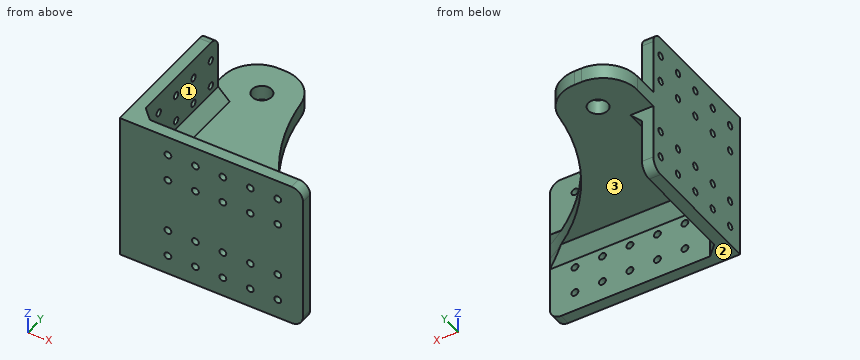
```python
from build123d import *

# Parameters (mm, degrees)
BOSS_EXTRU_1_DEPTH           = 65
ESQUISSE2_W                  = 80
ESQUISSE2_H                  = 6.5
BOSS_EXTRU_2_DEPTH           = 81
ENL_V_MAT_EXTRU_1_DEPTH      = 123.776473724
ENL_V_MAT_EXTRU_1_DEPTH_BACK = 123.776473724
CONG_1_R                     = 15
ENL_V_MAT_EXTRU_2_DEPTH      = 123.776473724
ENL_V_MAT_EXTRU_2_DEPTH_BACK = 123.776473724
ESQUISSE4_R                  = 4.25
CHANFREIN1_SIZE              = 5
ENL_V_MAT_EXTRU_3_DEPTH      = 135.242318216
ENL_V_MAT_EXTRU_3_DEPTH_BACK = 135.242318216
ESQUISSE5_R                  = 1.5
CONG_2_R                     = 5
ENL_V_MAT_EXTRU_4_DEPTH      = 135.242318216
ENL_V_MAT_EXTRU_4_DEPTH_BACK = 135.242318216
ESQUISSE6_R                  = 1.5


with BuildPart() as part:
    # Esquisse1 → Boss.-Extru.1 (new body)
    with BuildSketch(Plane.XY):
        Polygon((0, 0), (80, 0), (80, 5), (5, 5), (5, 60), (0, 60), align=None)
    extrude(amount=BOSS_EXTRU_1_DEPTH)

    # Esquisse2 → Boss.-Extru.2 (add)
    with BuildSketch(Plane(origin=(0, 5, 0), x_dir=(1, 0, 0), z_dir=(0, 1, 0))):
        with Locations((40, -32.5)):
            Rectangle(ESQUISSE2_W, ESQUISSE2_H)
    extrude(amount=BOSS_EXTRU_2_DEPTH)

    # Esquisse3 → Enlèv. mat.-Extru.1 (cut, two sides: drawn at the far end of the back side and taken through both)
    with BuildSketch(Plane.XY.offset(35.75).offset(-ENL_V_MAT_EXTRU_1_DEPTH_BACK)):
        with BuildLine():
            Line((32, 86), (80, 86))
            Line((80, 86), (80, 5))
            ThreePointArc((80, 5), (44.901203691, 38.922935521), (32, 86))
        make_face()
    extrude(amount=ENL_V_MAT_EXTRU_1_DEPTH + ENL_V_MAT_EXTRU_1_DEPTH_BACK, mode=Mode.SUBTRACT)

    # Congé1
    cong_1_edges = [part.edges().sort_by_distance(p)[0] for p in [
        (0, 86, 32.5),
        (32, 86, 32.5),
    ]]
    fillet(cong_1_edges, radius=CONG_1_R)

    # Esquisse4 → Enlèv. mat.-Extru.2 (cut, two sides: drawn at the far end of the back side and taken through both)
    with BuildSketch(Plane.XY.offset(35.75).offset(-ENL_V_MAT_EXTRU_2_DEPTH_BACK)):
        with Locations((17.5, 70.5)):
            Circle(ESQUISSE4_R)
    extrude(amount=ENL_V_MAT_EXTRU_2_DEPTH + ENL_V_MAT_EXTRU_2_DEPTH_BACK, mode=Mode.SUBTRACT)

    # Chanfrein1
    # the kernel refuses this chamfer: 5 mm, written as the material it adds along each edge
    with BuildSketch(Plane(origin=(8.333333333, 8.333333333, 39.083333333), x_dir=(0, 0.7071067811865474, -0.7071067811865476), z_dir=(-0.5773502691896261, -0.5773502691896257, -0.5773502691896255))) as chanfrein1_piece_1_section:
        Polygon((-3.535533906, 2.041241452), (3.535533906, 2.041241452), (0, -4.082482905), align=None)
    chanfrein1_piece_1 = extrude(amount=6.350852961, mode=Mode.PRIVATE)
    chanfrein1_piece_1 = split(chanfrein1_piece_1, bisect_by=Plane(origin=(5, 5, 35.75), z_dir=(0, 1, 0)), keep=Keep.TOP, mode=Mode.PRIVATE)
    chanfrein1_piece_1 = split(chanfrein1_piece_1, bisect_by=Plane(origin=(5, 5, 35.75), z_dir=(0, 0, 1)), keep=Keep.TOP, mode=Mode.PRIVATE)
    chanfrein1_piece_1 = split(chanfrein1_piece_1, bisect_by=Plane(origin=(5, 5, 35.75), z_dir=(1, 0, 0)), keep=Keep.TOP, mode=Mode.PRIVATE)
    add(chanfrein1_piece_1)
    with BuildSketch(Plane(origin=(8.333333333, 8.333333333, 25.916666667), x_dir=(0, -0.7071067811865474, -0.7071067811865476), z_dir=(-0.577350269189626, -0.5773502691896256, 0.5773502691896257))) as chanfrein1_piece_2_section:
        Polygon((-3.535533906, 2.041241452), (3.535533906, 2.041241452), (0, -4.082482905), align=None)
    chanfrein1_piece_2 = extrude(amount=6.350852961, mode=Mode.PRIVATE)
    chanfrein1_piece_2 = split(chanfrein1_piece_2, bisect_by=Plane(origin=(5, 5, 29.25), z_dir=(0, 0, -1)), keep=Keep.TOP, mode=Mode.PRIVATE)
    chanfrein1_piece_2 = split(chanfrein1_piece_2, bisect_by=Plane(origin=(5, 5, 29.25), z_dir=(0, 1, 0)), keep=Keep.TOP, mode=Mode.PRIVATE)
    chanfrein1_piece_2 = split(chanfrein1_piece_2, bisect_by=Plane(origin=(5, 5, 29.25), z_dir=(1, 0, 0)), keep=Keep.TOP, mode=Mode.PRIVATE)
    add(chanfrein1_piece_2)
    with BuildSketch(Plane(origin=(5, 5, 22.89158506), x_dir=(-0.027495876610586324, 0.9996219169112968, 0), z_dir=(0, 0, 1))) as chanfrein1_piece_3:
        Polygon((CHANFREIN1_SIZE * 0.999621916911, -CHANFREIN1_SIZE * 0.0274958766106), (-CHANFREIN1_SIZE * 0.0274958766106, -CHANFREIN1_SIZE * 0.999621916911), (0, 0), align=None)
    extrude(amount=42.10841494)
    with BuildSketch(Plane(origin=(5, 5, 0), x_dir=(0.9996219169112968, -0.02749587661058617, 0), z_dir=(0, 0, 1))) as chanfrein1_piece_4:
        Polygon((CHANFREIN1_SIZE * 0.999621916911, CHANFREIN1_SIZE * 0.0274958766106), (-CHANFREIN1_SIZE * 0.0274958766106, CHANFREIN1_SIZE * 0.999621916911), (0, 0), align=None)
    extrude(amount=42.10841494)
    with BuildSketch(Plane(origin=(5, 5, 35.75), x_dir=(0.9996219169112968, 0, -0.027495876610586327), z_dir=(0, 1, 0)), Plane(origin=(5, 60, 29.25), x_dir=(0.9996219169112968, 0, 0.027495876610586313), z_dir=(0, -1, 0))) as chanfrein1_piece_5:
        Polygon((CHANFREIN1_SIZE * 0.999621916911, -CHANFREIN1_SIZE * 0.0274958766106), (-CHANFREIN1_SIZE * 0.0274958766106, -CHANFREIN1_SIZE * 0.999621916911), (0, 0), align=None)
    extrude(amount=55)
    with BuildSketch(Plane(origin=(92.85841494, 5, 35.75), x_dir=(0, 0.9996219169112968, -0.027495876610586327), z_dir=(-1, 0, 0))) as chanfrein1_piece_6_section:
        Polygon((CHANFREIN1_SIZE * 0.999621916911, -CHANFREIN1_SIZE * 0.0274958766106), (-CHANFREIN1_SIZE * 0.0274958766106, -CHANFREIN1_SIZE * 0.999621916911), (0, 0), align=None)
    chanfrein1_piece_6 = extrude(amount=87.85841494, mode=Mode.PRIVATE)
    chanfrein1_piece_6 = chanfrein1_piece_6 - Plane(origin=(124.34375, 86, 37.432610037), x_dir=(-0.4802030456852788, -0.8771573604060916, 0), z_dir=(0, 0, -1)) * Cylinder(92.34375, 196, mode=Mode.PRIVATE)
    add(chanfrein1_piece_6)
    with BuildSketch(Plane(origin=(5, 5, 29.25), x_dir=(0, 0.9996219169112968, 0.027495876610586324), z_dir=(1, 0, 0))) as chanfrein1_piece_7_section:
        Polygon((CHANFREIN1_SIZE * 0.999621916911, -CHANFREIN1_SIZE * 0.0274958766106), (-CHANFREIN1_SIZE * 0.0274958766106, -CHANFREIN1_SIZE * 0.999621916911), (0, 0), align=None)
    chanfrein1_piece_7 = extrude(amount=87.85841494, mode=Mode.PRIVATE)
    chanfrein1_piece_7 = chanfrein1_piece_7 - Plane(origin=(124.34375, 86, 27.567389963), x_dir=(-0.4802030456852788, -0.8771573604060916, 0), z_dir=(0, 0, -1)) * Cylinder(92.34375, 196, mode=Mode.PRIVATE)
    add(chanfrein1_piece_7)

    # Esquisse5 → Enlèv. mat.-Extru.3 (cut, two sides: drawn at the far end of the back side and taken through both)
    with BuildSketch(Plane.ZY.offset(-ENL_V_MAT_EXTRU_3_DEPTH_BACK)):
        with Locations(Location((8.5, 55, 0), (0, 0, 270))):
            Circle(ESQUISSE5_R)
        with Locations(Location((8.5, 43, 0), (0, 0, 270))):
            Circle(ESQUISSE5_R)
        with Locations(Location((8.5, 31, 0), (0, 0, 270))):
            Circle(ESQUISSE5_R)
        with Locations(Location((20.5, 31, 0), (0, 0, 270))):
            Circle(ESQUISSE5_R)
        with Locations(Location((20.5, 43, 0), (0, 0, 270))):
            Circle(ESQUISSE5_R)
        with Locations(Location((20.5, 55, 0), (0, 0, 270))):
            Circle(ESQUISSE5_R)
        with Locations(Location((20.5, 7, 0), (0, 0, 90))):
            Circle(ESQUISSE5_R)
        with Locations(Location((20.5, 19, 0), (0, 0, 270))):
            Circle(ESQUISSE5_R)
        with Locations(Location((8.5, 19, 0), (0, 0, 270))):
            Circle(ESQUISSE5_R)
        with Locations(Location((8.5, 7, 0), (0, 0, 90))):
            Circle(ESQUISSE5_R)
        with Locations(Location((56.5, 7, 0), (0, 0, 90))):
            Circle(ESQUISSE5_R)
        with Locations(Location((56.5, 19, 0), (0, 0, 270))):
            Circle(ESQUISSE5_R)
        with Locations(Location((44.5, 19, 0), (0, 0, 270))):
            Circle(ESQUISSE5_R)
        with Locations(Location((44.5, 7, 0), (0, 0, 90))):
            Circle(ESQUISSE5_R)
        with Locations(Location((44.5, 55, 0), (0, 0, 270))):
            Circle(ESQUISSE5_R)
        with Locations(Location((44.5, 43, 0), (0, 0, 270))):
            Circle(ESQUISSE5_R)
        with Locations(Location((44.5, 31, 0), (0, 0, 270))):
            Circle(ESQUISSE5_R)
        with Locations(Location((56.5, 31, 0), (0, 0, 270))):
            Circle(ESQUISSE5_R)
        with Locations(Location((56.5, 43, 0), (0, 0, 270))):
            Circle(ESQUISSE5_R)
        with Locations(Location((56.5, 55, 0), (0, 0, 270))):
            Circle(ESQUISSE5_R)
    extrude(amount=ENL_V_MAT_EXTRU_3_DEPTH + ENL_V_MAT_EXTRU_3_DEPTH_BACK, mode=Mode.SUBTRACT)

    # Congé2
    cong_2_edges = [part.edges().sort_by_distance(p)[0] for p in [
        (80, 2.5, 65),
        (2.5, 60, 65),
        (2.5, 60, 0),
        (80, 2.5, 0),
    ]]
    fillet(cong_2_edges, radius=CONG_2_R)

    # Esquisse6 → Enlèv. mat.-Extru.4 (cut, two sides: drawn at the far end of the back side and taken through both)
    with BuildSketch(Plane.XZ.offset(-ENL_V_MAT_EXTRU_4_DEPTH_BACK)):
        with Locations((45, 56.5)):
            Circle(ESQUISSE6_R)
        with Locations((57, 56.5)):
            Circle(ESQUISSE6_R)
        with Locations((69, 56.5)):
            Circle(ESQUISSE6_R)
        with Locations((21, 56.5)):
            Circle(ESQUISSE6_R)
        with Locations((33, 56.5)):
            Circle(ESQUISSE6_R)
        with Locations((33, 44.5)):
            Circle(ESQUISSE6_R)
        with Locations((21, 44.5)):
            Circle(ESQUISSE6_R)
        with Locations((69, 44.5)):
            Circle(ESQUISSE6_R)
        with Locations((57, 44.5)):
            Circle(ESQUISSE6_R)
        with Locations((45, 44.5)):
            Circle(ESQUISSE6_R)
        with Locations((45, 20.5)):
            Circle(ESQUISSE6_R)
        with Locations((57, 20.5)):
            Circle(ESQUISSE6_R)
        with Locations((69, 20.5)):
            Circle(ESQUISSE6_R)
        with Locations((21, 20.5)):
            Circle(ESQUISSE6_R)
        with Locations((33, 20.5)):
            Circle(ESQUISSE6_R)
        with Locations((33, 8.5)):
            Circle(ESQUISSE6_R)
        with Locations((21, 8.5)):
            Circle(ESQUISSE6_R)
        with Locations((69, 8.5)):
            Circle(ESQUISSE6_R)
        with Locations((57, 8.5)):
            Circle(ESQUISSE6_R)
        with Locations((45, 8.5)):
            Circle(ESQUISSE6_R)
    extrude(amount=ENL_V_MAT_EXTRU_4_DEPTH + ENL_V_MAT_EXTRU_4_DEPTH_BACK, mode=Mode.SUBTRACT)


solid = part.part
```
Source: CAD feature listing. Evaluate the final solid. Frame: model axes, mm. Face numbers are marked on the shaded views. A direction names the side the tool comes from. Give positions to 0.01 mm unless a question says otherwise; leave off trailing zeros. Write each loop counter-clockwise with the first axis right and the second up, starting at its lowest first coordinate (ties: lowest second). Pieces come first, ordered by that corner, then holes.
1. Section query C-C (z = 32.5). Return the cut outline in (x, y).
2. Section query D-D (z = 44.5). Count the separate pieces of the cut face and the enclosed holes in it, then the cut area to 4 significant figures.
3. Access query for the marked faces 1, 2 and 3. Directions: +Z, -Z, +X, -X, +Y, -Y. A direction counts if a zero-diameter tool reaches every point of the face in a straight line with its end or side. Return the directions, or none.
4. First-contact query: pin 1 (7.5 mm diameter, centred on y = 45, z = 54, fed in from +X); pin 2 (5 mm diameter, centred on x = 34, y = 25, fed in from +Z); pin 3 (4 mm diameter, centred on y = 43, z = 56.5, fed in from -X); pin 4 (8 mm diameter, centred on x = 42, y = 37.5, fed in from -Z). Flat tips, straight axial feed; report the tip coordinate or a pass-through.
5. Section query B-B (x = 45). Return the cut outline in (y, z).
6. Section query A-A (y = 43). Return the cut outline in (x, z).
7. Material intervals for line 1 along Z through (x, y) = (2.05, 55); line 2 along X through (y, z) = (2.85, 20.5); line 3 along Y through (x, z) = (2.5, 44.5), sorted ascending.
Output values:
1. outline: (0, 0) - (80, 0) - (80, 5) arc R92.34 cw to (32.91, 73.1) arc R15 ccw to (18.05, 86) - (15, 86) arc R15 ccw to (0, 71) - close; hole circle Ø8.5 at (17.5, 70.5)
2. separate pieces: 11
2. enclosed holes: 0
2. area: 528.5 mm2
3. face 1: +Z, +X, +Y
3. face 2: -Z, +X, -X, +Y, -Y
3. face 3: -Z, +X, +Y
4. pin 1: stops at x = 5
4. pin 2: stops at z = 35.75
4. pin 3: stops at x = 0
4. pin 4: stops at z = 29.25
5. outline: (0, 0) - (5, 0) - (5, 7) - (0, 7) - close; (0, 10) - (5, 10) - (5, 19) - (0, 19) - close; (0, 22) - (5, 22) - (5, 24.25) - (10, 29.25) - (38.76, 29.25) - (38.76, 35.75) - (10, 35.75) - (5, 40.75) - (5, 43) - (0, 43) - close; (0, 46) - (5, 46) - (5, 55) - (0, 55) - close; (0, 58) - (5, 58) - (5, 65) - (0, 65) - close
6. outline: (0, 0) - (5, 0) - (5, 7) - (0, 7) - close; (0, 10) - (5, 10) - (5, 19) - (0, 19) - close; (0, 22) - (5, 22) - (5, 24.25) - (10, 29.25) - (42.62, 29.25) - (42.62, 35.75) - (10, 35.75) - (5, 40.75) - (5, 43) - (0, 43) - close; (0, 46) - (5, 46) - (5, 55) - (0, 55) - close; (0, 58) - (5, 58) - (5, 65) - (0, 65) - close
7. line 1: z = 0 to 7, 10 to 19, 22 to 43, 46 to 55, 58 to 65
7. line 2: x = 0 to 19.5, 22.5 to 31.5, 34.5 to 43.5, 46.5 to 55.5, 58.5 to 67.5, 70.5 to 80
7. line 3: y = 0 to 5.5, 8.5 to 17.5, 20.5 to 29.5, 32.5 to 41.5, 44.5 to 53.5, 56.5 to 60
